from build123d import *

# Parameters (mm, degrees)
F1_DEPTH = 50.8
F2_R     = 3.625658
F3_DEPTH = 50.8
F5_DEPTH = 44.45
F6_DEPTH = 38.1
F7_DEPTH = 12.7
F8_DEPTH = 6.35


with BuildPart() as f1:
    # F0 (on Top) → F1 (new body)
    with BuildSketch(Plane.XY):
        with BuildLine():
            Line((59.092954, 44.097524), (-50.835285, 44.097524))
            Line((-50.835285, 44.097524), (-50.835285, -43.112647))
            Line((-50.835285, -43.112647), (59.092954, -43.112647))
            Line((59.092954, -43.112647), (59.092954, -34.318248))
            ThreePointArc((59.092954, -34.318248), (24.774705, 0), (59.092954, 34.318248))
            Line((59.092954, 34.318248), (59.092954, 44.097524))
        make_face()
    extrude(amount=F1_DEPTH)

    # F2 (on face) → F3 (cut)
    with BuildSketch(Plane(origin=(-50.835285, 0, 0), x_dir=(0, -1, 0), z_dir=(-1, 0, 0))):
        with Locations((0, 24.232104)):
            Circle(F2_R)
    extrude(amount=-F3_DEPTH, mode=Mode.SUBTRACT)

    # F4 (on face) → F5 (cut)
    with BuildSketch(Plane.XY.offset(50.8)):
        with BuildLine():
            ThreePointArc((59.092954, -39.50878), (19.584174, 0), (59.092954, 39.50878))
            Line((59.092954, 39.50878), (59.092954, 42.25664))
            ThreePointArc((59.092954, 42.25664), (16.836314, 0), (59.092954, -42.25664))
            Line((59.092954, -42.25664), (59.092954, -39.50878))
        make_face()
    extrude(amount=-F5_DEPTH, mode=Mode.SUBTRACT)

    # F4 (on face) → F6 (join)
    with BuildSketch(Plane.XY.offset(50.8)):
        with BuildLine():
            ThreePointArc((59.092954, -39.50878), (19.584174, 0), (59.092954, 39.50878))
            Line((59.092954, 39.50878), (59.092954, 42.25664))
            ThreePointArc((59.092954, 42.25664), (16.836314, 0), (59.092954, -42.25664))
            Line((59.092954, -42.25664), (59.092954, -39.50878))
        make_face()
    extrude(amount=-F6_DEPTH)

    # F4 (on face) → F7 (cut)
    with BuildSketch(Plane.XY.offset(50.8)):
        with BuildLine():
            ThreePointArc((59.092954, -39.50878), (19.584174, 0), (59.092954, 39.50878))
            Line((59.092954, 39.50878), (59.092954, 42.25664))
            ThreePointArc((59.092954, 42.25664), (16.836314, 0), (59.092954, -42.25664))
            Line((59.092954, -42.25664), (59.092954, -39.50878))
        make_face()
    extrude(amount=-F7_DEPTH, mode=Mode.SUBTRACT)

    # F4 (on face) → F8 (join)
    with BuildSketch(Plane.XY.offset(50.8)):
        with BuildLine():
            ThreePointArc((59.092954, -39.50878), (19.584174, 0), (59.092954, 39.50878))
            Line((59.092954, 39.50878), (59.092954, 42.25664))
            ThreePointArc((59.092954, 42.25664), (16.836314, 0), (59.092954, -42.25664))
            Line((59.092954, -42.25664), (59.092954, -39.50878))
        make_face()
    extrude(amount=-F8_DEPTH)


solid = f1.part
Check sheet for the modelled part. Datum: model origin and axes. Units: mm. A direction names the side the tool comes from. Give positions to 0.01 mm unless a question says otherwise; leave off trailing zeros. Write each loop counter-clockwise with the first axis right and the second up, starting at its lowest first coordinate (ties: lowest second). Pieces come first, ordered by that corner, then holes. Notation, with made-up numbers: (2, 25) -> (49, 25) arc R24 ccw to (49, 39) -> close; hole circle Ø10 at (16, 58.25). An arc over 180 degrees is marked (long way). Use one line per item in the form item = value. Start each with the question number.
1. Section check A-A (z = 40). Record the cut outline in (x, y), and give its area (3 significant figures).
2. Section check D-D (y = -22.5). Record the cut outline in (x, z), and give its area (3 significant figures).
3. Go/stop test with flat-tipped pins: P1, Ø2, axis at y = -1.5, z = 22.5, coming from the -X side; P2, Ø10, axis at y = 19, z = 29.5, coming from the +X side. Record where each tip stops, or that it passes through.
4. Section check B-B (y = 0). Record the cut outline in (x, z).
5. Thickness scan on line 1 along Z through (x, y) = (-10.5, 0); line 2 along X through (y, z) = (0, 8); line 3 along X through (y, z) = (29.5, 41.5). Record the ranges inside material, lowest first. Write a range as from..to.
6. Section check C-C (z = 32). Record the cut outline in (x, y).
7. Mould release check, pull along X, two halves, no side actions. Record for faces 1 (the cylindrical face through (24.783, -0.755, 25.044)), 2 (the flat face through (19, 0, 12.7)), 3 (the cylindrical face through (16.847, 0.929, 41.319)), 4 (the flat face through (-9, 1, 50.8)): pulls with the +X half, pulls with the -X half, needs draft (parallel to the pull), parting line crosses it, or undercut.
8. Access from +Z, -Z, +X, -X, +Y, -Y to the whole of each face (thin tool, end or side, straight path). Record for faces 5 (the flat face through (19, 0, 6.35)), 6 (the flat face through (59.093, 39, 26)), 7 (the flat face through (-0.035, 0, 24)).
Conclusion:
q1.outline = (-50.84, -43.11) -> (59.09, -43.11) -> (59.09, -42.26) arc R42.26 cw to (59.09, 42.26) -> (59.09, 44.1) -> (-50.84, 44.1) -> close; (59.09, -39.51) -> (59.09, -34.32) arc R34.32 cw to (59.09, 34.32) -> (59.09, 39.51) arc R39.51 ccw to start
q1.area = 7,380 mm²
q2.outline = (-50.84, 0) -> (33.18, 0) -> (33.18, 50.8) -> (-50.84, 50.8) -> close; hole (23.32, 6.35) -> (26.62, 6.35) -> (26.62, 12.7) -> (23.32, 12.7) -> close; hole (23.32, 38.1) -> (26.62, 38.1) -> (26.62, 44.45) -> (23.32, 44.45) -> close
q2.area = 4,230 mm²
q3.P1 = -0.04
q3.P2 = 34.56
q4.outline = (-50.84, 0) -> (24.77, 0) -> (24.77, 50.8) -> (-50.84, 50.8) -> (-50.84, 27.86) -> (-0.04, 27.86) -> (-0.04, 20.61) -> (-50.84, 20.61) -> close; hole (16.84, 6.35) -> (19.58, 6.35) -> (19.58, 12.7) -> (16.84, 12.7) -> close; hole (16.84, 38.1) -> (19.58, 38.1) -> (19.58, 44.45) -> (16.84, 44.45) -> close
q5.line_1 = 0..20.61, 27.86..50.8
q5.line_2 = -50.84..16.84, 19.58..24.77
q5.line_3 = -50.84..28.84, 32.81..41.56
q6.outline = (-50.84, -43.11) -> (59.09, -43.11) -> (59.09, -34.32) arc R34.32 cw to (59.09, 34.32) -> (59.09, 44.1) -> (-50.84, 44.1) -> close
q7.face_1 = pulls with the +X half
q7.face_2 = undercut
q7.face_3 = undercut
q7.face_4 = needs draft
q8.face_5 = none
q8.face_6 = +Z, -Z, +X, +Y, -Y
q8.face_7 = -X
